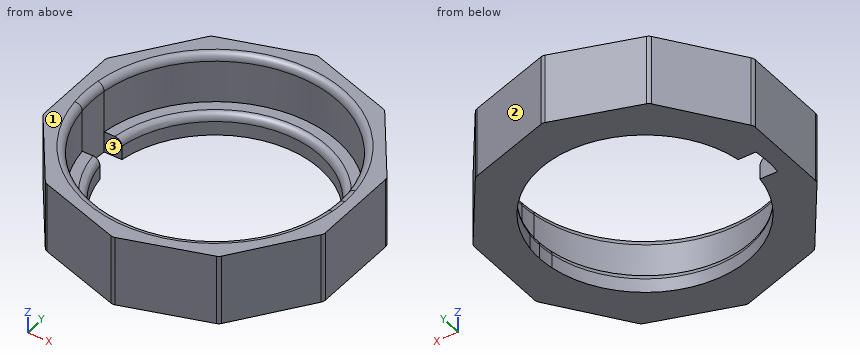
```python
from build123d import *

# Parameters (mm, degrees)
F1_DEPTH = 10
F2_DEPTH = 3
F3_R     = 1
F4_R     = 1
F5_R     = 1


with BuildPart() as f1:
    # F0 (on Top) → F1 (new body)
    with BuildSketch(Plane.XY):
        with BuildLine():
            ThreePointArc((17.3547543918, 2.25), (17.4636508476, 1.1273415949), (17.5, 0))
            ThreePointArc((17.5, 0), (17.4636508476, -1.1273415949), (17.3547543918, -2.25))
            Line((17.3547543918, -2.25), (20.0049429916, -2.25))
            Line((20.0049429916, -2.25), (20.0049429916, 2.25))
            Line((20.0049429916, 2.25), (17.3547543918, 2.25))
        make_face()
        with BuildLine():
            ThreePointArc((-17.3547543918, 2.25), (0, 17.5), (17.3547543918, 2.25))
            Line((17.3547543918, 2.25), (20.0049429916, 2.25))
            Line((20.0049429916, 2.25), (20.0049429916, 6.5))
            Line((20.0049429916, 6.5), (12.3637347118, 17.0172209269))
            Line((12.3637347118, 17.0172209269), (0, 21.0344418537))
            Line((0, 21.0344418537), (-12.3637347118, 17.0172209269))
            Line((-12.3637347118, 17.0172209269), (-20.0049429916, 6.5))
            Line((-20.0049429916, 6.5), (-20.0049429916, 2.25))
            Line((-20.0049429916, 2.25), (-17.3547543918, 2.25))
        make_face()
        with BuildLine():
            Line((20.0049429916, -2.25), (17.3547543918, -2.25))
            ThreePointArc((17.3547543918, -2.25), (0, -17.5), (-17.3547543918, -2.25))
            Line((-17.3547543918, -2.25), (-20.0049429916, -2.25))
            Line((-20.0049429916, -2.25), (-20.0049429916, -6.5))
            Line((-20.0049429916, -6.5), (-12.3637347118, -17.0172209269))
            Line((-12.3637347118, -17.0172209269), (0, -21.0344418537))
            Line((0, -21.0344418537), (12.3637347118, -17.0172209269))
            Line((12.3637347118, -17.0172209269), (20.0049429916, -6.5))
            Line((20.0049429916, -6.5), (20.0049429916, -2.25))
        make_face()
        with BuildLine():
            ThreePointArc((-17.3547543918, -2.25), (-17.5, 0), (-17.3547543918, 2.25))
            Line((-17.3547543918, 2.25), (-20.0049429916, 2.25))
            Line((-20.0049429916, 2.25), (-20.0049429916, -2.25))
            Line((-20.0049429916, -2.25), (-17.3547543918, -2.25))
        make_face()
    extrude(amount=F1_DEPTH)

    # F0 (on Top) → F2 (join)
    with BuildSketch(Plane.XY):
        with BuildLine():
            ThreePointArc((17.3547543918, -2.25), (17.4636508476, -1.1273415949), (17.5, 0))
            ThreePointArc((17.5, 0), (17.4636508476, 1.1273415949), (17.3547543918, 2.25))
            Line((17.3547543918, 2.25), (14.83028995, 2.25))
            ThreePointArc((14.83028995, 2.25), (14.957512314, 1.1281956281), (15, 0))
            ThreePointArc((15, 0), (14.957512314, -1.1281956281), (14.83028995, -2.25))
            Line((14.83028995, -2.25), (17.3547543918, -2.25))
        make_face()
        with BuildLine():
            ThreePointArc((-17.3547543918, -2.25), (0, -17.5), (17.3547543918, -2.25))
            Line((17.3547543918, -2.25), (14.83028995, -2.25))
            ThreePointArc((14.83028995, -2.25), (0, -15), (-14.83028995, -2.25))
            Line((-14.83028995, -2.25), (-17.3547543918, -2.25))
        make_face()
        with BuildLine():
            Line((14.83028995, 2.25), (17.3547543918, 2.25))
            ThreePointArc((17.3547543918, 2.25), (0, 17.5), (-17.3547543918, 2.25))
            Line((-17.3547543918, 2.25), (-14.83028995, 2.25))
            ThreePointArc((-14.83028995, 2.25), (0, 15), (14.83028995, 2.25))
        make_face()
    extrude(amount=F2_DEPTH)

    # F3
    f3_edges = [f1.edges().sort_by_distance(p)[0] for p in [
        (15, 0, 3),
    ]]
    fillet(f3_edges, radius=F3_R)

    # F4
    f4_edges = [f1.edges().sort_by_distance(p)[0] for p in [
        (20.004943, -6.5, 5),
        (12.363735, -17.017221, 5),
        (0, -21.034442, 5),
        (-12.363735, -17.017221, 5),
        (-20.004943, -6.5, 5),
        (-20.004943, 6.5, 5),
        (0, 21.034442, 5),
        (-12.363735, 17.017221, 5),
        (12.363735, 17.017221, 5),
        (20.004943, 6.5, 5),
    ]]
    fillet(f4_edges, radius=F4_R)

    # F5
    f5_edges = [f1.edges().sort_by_distance(p)[0] for p in [
        (17.354754, 2.25, 10),
    ]]
    fillet(f5_edges, radius=F5_R)


solid = f1.part
```
For this review, take the finished solid that the model builds, in its own axes (mm). Face numbers are marked on the shaded views. Round coordinates to 2 decimals unless told otherwise and drop trailing zeros. Order: outer loops, then holes, each group sorted by start corner. A loop starts at its lowest first (then second) coordinate and runs counter-clockwise, first axis right, second up. Notation, with made-up numbers: (-28.75, 57) -> (-19.75, 57) arc R20 ccw to (-19.75, 83) -> close; hole circle Ø4 at (19.25, 48). An arc over 180 degrees is marked (long way). Use a Markdown table: item, result.
Item 1: Take a section at B-B (z = 2.5). State the section outline as (x, y) points.
Resolved:
| item | result |
|---|---|
| outline | (-20, -6.18) arc R1 ccw to (-19.81, -6.76) -> (-12.55, -16.75) arc R1 ccw to (-12.05, -17.12) -> (-0.31, -20.93) arc R1 ccw to (0.31, -20.93) -> (12.05, -17.12) arc R1 ccw to (12.55, -16.75) -> (19.81, -6.76) arc R1 ccw to (20, -6.18) -> (20, 6.18) arc R1 ccw to (19.81, 6.76) -> (12.55, 16.75) arc R1 ccw to (12.05, 17.12) -> (0.31, 20.93) arc R1 ccw to (-0.31, 20.93) -> (-12.05, 17.12) arc R1 ccw to (-12.55, 16.75) -> (-19.81, 6.76) arc R1 ccw to (-20, 6.18) -> close; hole (-17.35, -2.25) -> (-14.97, -2.25) arc R15.13 ccw (long way) to (-14.97, 2.25) -> (-17.35, 2.25) arc R17.5 ccw to start |
Item 2: For pin 1 (2 mm diameter, centred on x = 8.5, z = 3, fed in from +Y); pin 2 (4 mm diameter, centred on y = -10, z = 7, fed in from -X); pin 3 (0.8 mm diameter, centred on x = -16.5, z = 2, fed in from -Y), all flat-tipped, find the tip position at first contact; note any pin that passes through.
Resolved:
| item | result |
|---|---|
| pin 1 | stops at y = 18.6 |
| pin 2 | stops at x = -18.92 |
| pin 3 | stops at y = -11.87 |
Item 3: Take a section at A-A (z = 6). State the section outline as (x, y) points.
Resolved:
| item | result |
|---|---|
| outline | (-20, -6.18) arc R1 ccw to (-19.81, -6.76) -> (-12.55, -16.75) arc R1 ccw to (-12.05, -17.12) -> (-0.31, -20.93) arc R1 ccw to (0.31, -20.93) -> (12.05, -17.12) arc R1 ccw to (12.55, -16.75) -> (19.81, -6.76) arc R1 ccw to (20, -6.18) -> (20, 6.18) arc R1 ccw to (19.81, 6.76) -> (12.55, 16.75) arc R1 ccw to (12.05, 17.12) -> (0.31, 20.93) arc R1 ccw to (-0.31, 20.93) -> (-12.05, 17.12) arc R1 ccw to (-12.55, 16.75) -> (-19.81, 6.76) arc R1 ccw to (-20, 6.18) -> close; hole circle Ø35 at (0, 0) |
Item 4: Draft analysis for pull direction Y (two halves, no side actions). For the marked faces 1, 2 and 3, state which applies: +Y half, -Y half, draft (parallel to the pull), parting line (faces both ways), or undercut.
Resolved:
| item | result |
|---|---|
| face 1 | draft |
| face 2 | +Y half |
| face 3 | undercut |
Item 5: For line 1 along Z through (x, y) = (9, 14); line 2 along Y through (x, z) = (-13.5, 9.5); line 3 along X through (y, z) = (13.5, 4.25), list the stretches that pass through material, from the lowest coordinate up. Write a range as [from, to].
Resolved:
| item | result |
|---|---|
| line 1 | z = [0, 3] |
| line 2 | y = [-15.45, -11.34], [11.34, 15.45] |
| line 3 | x = [-14.92, -11.14], [11.14, 14.92] |
